Build history of the part. All positions in model axes, mm. A direction names the side the tool comes from. Coordinates: 2 decimals unless noted, no trailing zeros. Order: outer loops, then holes, each group sorted by start corner. A loop starts at its lowest first (then second) coordinate and runs counter-clockwise, first axis right, second up. Notation, with made-up numbers: (32, -2) - (44, -2) arc R20 ccw to (44, 26) - close; hole circle Ø8 at (-1.5, 3.25). An arc over 180 degrees is marked (long way). Answer as CSV lines item,"result". Start each with the question number.
from build123d import *

# Parameters (mm, degrees)
SKETCH1_W           = 56
SKETCH1_H           = 31
BOSS_EXTRUDE1_DEPTH = 9
SKETCH2_W           = 27
SKETCH2_H           = 52
CUT_EXTRUDE1_DEPTH  = 65.637450445
SKETCH3_W           = 8
SKETCH3_H           = 52
BOSS_EXTRUDE2_DEPTH = 4


with BuildPart() as part:
    # Sketch1 → Boss-Extrude1 (new body)
    with BuildSketch(Plane(origin=(0, 0, 0), x_dir=(0, 1, 0), z_dir=(0, 0, 1))):
        with Locations((28, 15.5)):
            Rectangle(SKETCH1_W, SKETCH1_H)
    extrude(amount=BOSS_EXTRUDE1_DEPTH)

    # Sketch2 → Cut-Extrude1 (cut, through all)
    with BuildSketch(Plane.XY.offset(9)):
        with Locations((-15.5, 28)):
            Rectangle(SKETCH2_W, SKETCH2_H)
    extrude(amount=-CUT_EXTRUDE1_DEPTH, mode=Mode.SUBTRACT)

    # Sketch3 → Boss-Extrude2 (add)
    with BuildSketch(Plane.XY.offset(9)):
        with Locations((-16.433368265, 28)):
            Rectangle(SKETCH3_W, SKETCH3_H)
    extrude(amount=-BOSS_EXTRUDE2_DEPTH)


solid = part.part
(1) Pull direction Y, two halves, no side cores. Call faces 4 (the flat face through (-15, 56, 4)), 5 (the flat face through (0, 28, 4)), 6 (the flat face through (-15.7, 54, 4.6)): +Y half, -Y half, draft (parallel to the pull), parting line (faces both ways), or undercut.
(2) Which spindle directions (+Z, -Z, +X, -X, +Y, -Y) get a long thin tool onto all of the face, cutting with end or side? Do faces 1 (the flat face through (-2, 28, 5)), 2 (the flat face through (-15.7, 2, 4.6)), 3 (the flat face through (-1.8, 25.8, 0)). Say none if no direction does.
(3) Band-saw the part on A-A on y = 42.5. List the corners of the cut face in (x, z).
(4) Band-saw the part on B-B on x = -22.5. List the corners of the cut face in (y, z).
(5) Band-saw the part on D-D on x = -15. List the corners of the cut face in (y, z).
(6) Drop flat-ended pins along their axis: pin 1 Ø3 at (y, z) = (23.5, 7) entering from +X; pin 2 Ø2 at (x, y) = (-10, 41.5) entering from -Z; pin 3 Ø4 at (x, y) = (-18, 15.5) entering from -Z. Give the stop position or say it passes through.
(7) Probe L1, parallel to X at y = 22.5, z = 8; L2, parallel to X at y = 51, z = 4.75; L3, parallel to Y at x = -27.5, z = 7.5. List the from-to ranges inside material, lowest first. Write a range as [from, to].
(8) Band-saw the part on C-C on z = 2.25. List the corners of the cut face in (x, y), plus the area to 3 significant figures.
Filled in:
1,face 4,"+Y half"
1,face 5,"draft"
1,face 6,"undercut"
2,face 1,"+Z, -Z"
2,face 2,"-Z"
2,face 3,"-Z, +X, -X, +Y, -Y"
3,outline,"(-31, 0) - (-29, 0) - (-29, 9) - (-31, 9) - close; (-20.43, 5) - (-12.43, 5) - (-12.43, 9) - (-20.43, 9) - close; (-2, 0) - (0, 0) - (0, 9) - (-2, 9) - close"
4,outline,"(0, 0) - (2, 0) - (2, 9) - (0, 9) - close; (54, 0) - (56, 0) - (56, 9) - (54, 9) - close"
5,outline,"(0, 0) - (2, 0) - (2, 5) - (54, 5) - (54, 0) - (56, 0) - (56, 9) - (0, 9) - close"
6,pin 1,"stops at x = 0"
6,pin 2,"passes through"
6,pin 3,"stops at z = 5"
7,L1,"x = [-31, -29], [-20.43, -12.43], [-2, 0]"
7,L2,"x = [-31, -29], [-2, 0]"
7,L3,"y = [0, 2], [54, 56]"
8,outline,"(-31, 0) - (0, 0) - (0, 56) - (-31, 56) - close; hole (-29, 2) - (-2, 2) - (-2, 54) - (-29, 54) - close"
8,area,"332 mm^2"
